The model under review builds one solid part; all positions refer to its coordinate system, in mm. A direction names the side the tool comes from. Give positions to 0.01 mm unless a question says otherwise; leave off trailing zeros. Order: outer loops, then holes, each group sorted by start corner. A loop starts at its lowest first (then second) coordinate and runs counter-clockwise, first axis right, second up. Notation, with made-up numbers: M 69.25,64 L 102.25,64 A18 ccw 102.25,92 Z; hole C 19,18 d5. An arc over 180 degrees is marked long. One line per question, with ' | ' between items. Start each with the question number.
1. The part is to be moulded in two halves that separate along Z. For faces 1 (the face through (-2, 2, 0)), 2 (the face through (7, 108, 895)), 3 (the face through (17, -12, 1420)), 4 (the face through (-171, -147, 1251)), say which applies: +Z half, -Z half, draft (parallel to the pull), parting line (faces both ways), or undercut.
2. Insertion check: P1, Ø12, axis at x = 9.5, z = 834, coming from the -Y side; P2, Ø15.5, axis at x = -2, z = 5.5, coming from the -Y side; P3, Ø6, axis at y = 87.5, z = 1088.5, coming from the +X side. Each pin has a flat end and moves straight along its axis. Give the tip position at first contact, or say it passes through.
3. We need section C-C on z = 1110. Write out the cut boundary in (x, y).
4. We need section A-A on x = 144. Write out the cut boundary in (y, z), then the cut area to 3 significant figures.
5. We need section B-B on y = -4.5. Write out the cut boundary in (x, z).
6. For faces 5 (the face through (-171, -147, 541)), 6 (the face through (7, -8, 374.5)), 7 (the face through (-2, -18, 355)), 8 (the face through (177.5, 113, 186)), list the 3-axis set-ups (+Z, -Z, +X, -X, +Y, -Y) from which the entire face can be reached by the end or side of a thin tool; tool diameter is ignored.
7. We need section D-D on z = 152.5. Write out the cut boundary in (x, y), then the cut area to 3 significant figures.
8. Wall thickness on L1, parallel to Z at x = -47, y = -9; L2, parallel to X at y = -44, z = 413; L3, parallel to Y at x = -141, z = 1444: over which ranges is each line inside the solid? List them lowest first.
```python
from build123d import *

# Parameters (mm, degrees)
F0_W      = 355
F0_H      = 255
F1_DEPTH  = 19.5
F2_W      = 355
F2_H      = 19.5
F3_DEPTH  = 355
F4_W      = 355
F4_H      = 19.5
F5_DEPTH  = 255
F6_W      = 19.5
F6_H      = 274.5
F7_DEPTH  = 355
F8_W      = 274.5
F8_H      = 19.5
F9_DEPTH  = 355
F10_W     = 374.5
F10_H     = 19.5
F11_DEPTH = 355
F12_W     = 374.5
F12_H     = 19.5
F13_DEPTH = 255
F14_W     = 19.5
F14_H     = 274.5
F15_DEPTH = 355
F16_W     = 274.5
F16_H     = 19.5
F17_DEPTH = 355
F18_W     = 374.5
F18_H     = 19.5
F19_DEPTH = 355
F20_W     = 374.5
F20_H     = 19.5
F21_DEPTH = 255


with BuildPart() as f1:
    # F0 (on Top) → F1 (new body)
    with BuildSketch(Plane.XY):
        Rectangle(F0_W, F0_H)
    extrude(amount=F1_DEPTH)

    # F2 (on face) → F3 (join)
    with BuildSketch(Plane.XY.offset(19.5)):
        with Locations((0, 117.75)):
            Rectangle(F2_W, F2_H)
    extrude(amount=F3_DEPTH)

    # F4 (on face) → F5 (join)
    with BuildSketch(Plane.XZ.offset(-108)):
        with Locations((0, 364.75)):
            Rectangle(F4_W, F4_H)
    extrude(amount=F5_DEPTH)

    # F6 (on face) → F7 (join)
    with BuildSketch(Plane.XY.offset(374.5)):
        with Locations((-167.75, -9.75)):
            Rectangle(F6_W, F6_H)
    extrude(amount=F7_DEPTH)

    # F8 (on face) → F9 (join)
    with BuildSketch(Plane.YZ.offset(-158)):
        with Locations((-9.75, 719.75)):
            Rectangle(F8_W, F8_H)
    extrude(amount=F9_DEPTH)

    # F10 (on face) → F11 (join)
    with BuildSketch(Plane.XY.offset(729.5)):
        with Locations((9.75, 117.75)):
            Rectangle(F10_W, F10_H)
    extrude(amount=F11_DEPTH)

    # F12 (on face) → F13 (join)
    with BuildSketch(Plane.XZ.offset(-108)):
        with Locations((9.75, 1074.75)):
            Rectangle(F12_W, F12_H)
    extrude(amount=F13_DEPTH)

    # F14 (on face) → F15 (join)
    with BuildSketch(Plane.XY.offset(1084.5)):
        with Locations((-167.75, -9.75)):
            Rectangle(F14_W, F14_H)
    extrude(amount=F15_DEPTH)

    # F16 (on face) → F17 (join)
    with BuildSketch(Plane.YZ.offset(-158)):
        with Locations((-9.75, 1429.75)):
            Rectangle(F16_W, F16_H)
    extrude(amount=F17_DEPTH)

    # F18 (on face) → F19 (join)
    with BuildSketch(Plane.XY.offset(1439.5)):
        with Locations((9.75, 117.75)):
            Rectangle(F18_W, F18_H)
    extrude(amount=F19_DEPTH)

    # F20 (on face) → F21 (join)
    with BuildSketch(Plane.XZ.offset(-108)):
        with Locations((9.75, 1784.75)):
            Rectangle(F20_W, F20_H)
    extrude(amount=F21_DEPTH)


solid = f1.part
```
Entries:
1) face 1: -Z half | face 2: undercut | face 3: undercut | face 4: draft
2) P1: stops at y = 108 | P2: stops at y = -127.5 | P3: stops at x = -158
3) outline: M -177.5,-147 L -158,-147 L -158,127.5 L -177.5,127.5 Z
4) outline: M -147,355 L 108,355 L 108,19.5 L -127.5,19.5 L -127.5,0 L 127.5,0 L 127.5,374.5 L -147,374.5 Z; M -147,710 L 127.5,710 L 127.5,1084.5 L -147,1084.5 L -147,1065 L 108,1065 L 108,729.5 L -147,729.5 Z; M -147,1420 L 127.5,1420 L 127.5,1794.5 L -147,1794.5 L -147,1775 L 108,1775 L 108,1439.5 L -147,1439.5 Z | area: 51,400 mm^2
5) outline: M -177.5,0 L 177.5,0 L 177.5,19.5 L -177.5,19.5 Z; M -177.5,355 L 177.5,355 L 177.5,374.5 L -158,374.5 L -158,710 L 197,710 L 197,729.5 L -177.5,729.5 Z; M -177.5,1065 L 197,1065 L 197,1084.5 L -158,1084.5 L -158,1420 L 197,1420 L 197,1439.5 L -177.5,1439.5 Z; M -177.5,1775 L 197,1775 L 197,1794.5 L -177.5,1794.5 Z
6) face 5: +Z, -Z, +X, -X, -Y | face 6: +X, +Y, -Y | face 7: +X, -X, -Y | face 8: -Z, +X, +Y, -Y
7) outline: M -177.5,108 L 177.5,108 L 177.5,127.5 L -177.5,127.5 Z | area: 6,920 mm^2
8) L1: z = 0 to 19.5, 355 to 374.5, 710 to 729.5, 1065 to 1084.5, 1420 to 1439.5, 1775 to 1794.5 | L2: x = -177.5 to -158 | L3: y = 108 to 127.5
